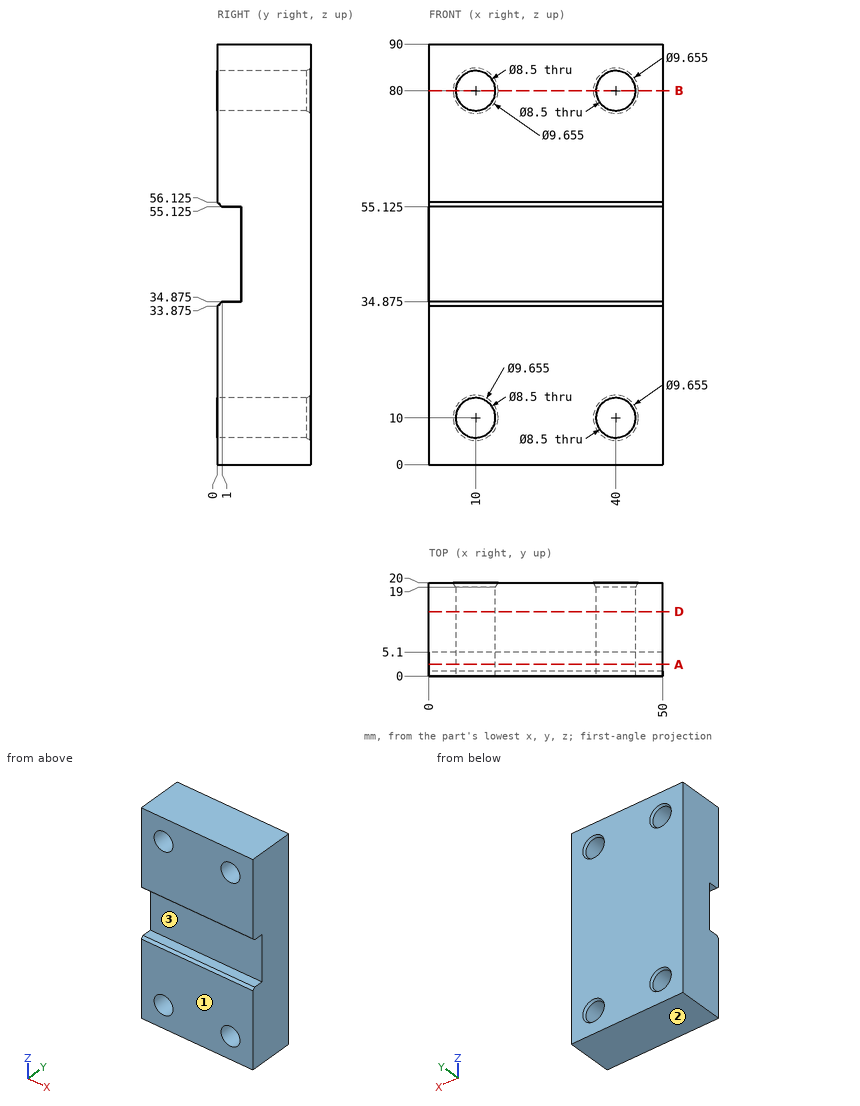
Check sheet for the drawn part. Datum: minimum x, y, z corner. Units: mm. Give positions to 0.01 mm unless a question says otherwise; leave off trailing zeros. Order: outer loops, then holes, each group sorted by start corner. A loop starts at its lowest first (then second) coordinate and runs counter-clockwise, first axis right, second up. Notation, with made-up numbers: (-33.5, 73) - (-21.5, 73) arc R15 ccw to (-21.5, 90) - close; hole circle Ø6 at (56.5, 54.5). An arc over 180 degrees is marked (long way). Answer as a JSON object with one key per item and string values.
(1) Cross-section at B-B (z = 80). Record the cut outline in (x, y), then the cut area to 3 significant figures.
Report:
{"outline": "(0, 0) - (5.75, 0) - (5.75, 19) - (5.17, 20) - (0, 20) - close; (14.25, 0) - (35.75, 0) - (35.75, 19) - (35.17, 20) - (14.83, 20) - (14.25, 19) - close; (44.25, 0) - (50, 0) - (50, 20) - (44.83, 20) - (44.25, 19) - close", "area": "659 mm^2"}
(2) Depth check by flat-ended pin: pin 1 Ø5 at (x, z) = (10, 10) entering from -Y; pin 2 Ø10 at (x, z) = (14.5, 48) entering from -Y. Enter the tip coordinate at first touch or a pass-through.
Report:
{"pin 1": "through", "pin 2": "y = 5.1"}
(3) Draft check along Z on the marked faces 1, 2 and 3. Enter one of: released by +Z, released by -Z, zero draft, split by the parting line, or undercut.
Report:
{"face 1": "zero draft", "face 2": "released by -Z", "face 3": "undercut"}
(4) Material ranges on line 1 (Z direction, x = 40, y = 8.5); line 2 (X direction, y = 8.25, z = 83); line 3 (Z direction, x = 39, y = 11), recorded low to high.
Report:
{"line 1": "0 to 5.75, 14.25 to 75.75, 84.25 to 90", "line 2": "0 to 6.99, 13.01 to 36.99, 43.01 to 50", "line 3": "0 to 5.87, 14.13 to 75.87, 84.13 to 90"}
(5) Cross-section at A-A (y = 2.5). State how many separate pieces and enclosed holes the cut face has, then the cut area to 3 significant figures.
Report:
{"separate pieces": "2", "enclosed holes": "4", "area": "3,260 mm^2"}
(6) Cross-section at D-D (y = 13.75). Record the cut outline in (x, z), then the cut area to 3 significant figures.
Report:
{"outline": "(0, 0) - (50, 0) - (50, 90) - (0, 90) - close; hole circle Ø8.5 at (10, 10); hole circle Ø8.5 at (10, 80); hole circle Ø8.5 at (40, 10); hole circle Ø8.5 at (40, 80)", "area": "4,270 mm^2"}
